```python
from build123d import *

# Parameters (mm, degrees)
SKETCH_1_R               = 27.65
SKETCH_1_R_2             = 17.65
EXTRUDE_1_DEPTH          = 167.37
CUT_EXTRUDE_1_DEPTH      = 20
CUT_EXTRUDE_START        = 147.37
CUT_EXTRUDE_2_DEPTH      = 20
CUT_EXTRUDE_4_DEPTH      = 26
CUT_EXTRUDE_4_DEPTH_BACK = 26
SKETCH_5_R               = 1.6
CUT_EXTRUDE_START_2      = 27.194163
CUT_EXTRUDE_3_DEPTH      = 2.45
CUT_EXTRUDE_5_DEPTH      = 2.45
CUT_EXTRUDE_START_3      = 27.2
CUT_EXTRUDE_6_DEPTH      = 2.45
PATTERN_CIRCULAR_2_COUNT = 4
SKETCH_8_R               = 1.6
CUT_EXTRUDE_7_DEPTH      = 32.4
PATTERN_CIRCULAR_3_COUNT = 4


with BuildPart() as part:
    # 草图1 → 凸台-拉伸1 (new body)
    with BuildSketch(Plane(origin=(0, 0, 0), x_dir=(1, 0, 0), z_dir=(0, 1, 0))):
        with Locations(Location((0, 0, 0), (0, 0, 270))):
            Circle(SKETCH_1_R)
        with Locations(Location((0, 0, 0), (0, 0, 270))):
            Circle(SKETCH_1_R_2, mode=Mode.SUBTRACT)
    extrude(amount=EXTRUDE_1_DEPTH)

    # 草图2 → 切除-拉伸1 (cut)
    with BuildSketch(Plane(origin=(0, 0, 0), x_dir=(1, 0, 0), z_dir=(0, 1, 0))):
        with BuildLine():
            Line((-27.194162977, 5), (-27.194162977, -5))
            ThreePointArc((-27.194162977, -5), (-27.65, 0), (-27.194162977, 5))
        make_face()
        with BuildLine():
            Line((27.194162977, -5), (27.194162977, 5))
            ThreePointArc((27.194162977, 5), (27.65, 0), (27.194162977, -5))
        make_face()
    extrude(amount=CUT_EXTRUDE_1_DEPTH, mode=Mode.SUBTRACT)

    # 草图3 → 切除-拉伸2 (cut)
    with BuildSketch(Plane(origin=(0, 0, 0), x_dir=(1, 0, 0), z_dir=(0, 1, 0)).offset(CUT_EXTRUDE_START)):
        with BuildLine():
            Line((-27.194162977, 5), (-27.194162977, -5))
            ThreePointArc((-27.194162977, -5), (-27.65, 0), (-27.194162977, 5))
        make_face()
        with BuildLine():
            Line((-5, -27.194162977), (5, -27.194162977))
            ThreePointArc((5, -27.194162977), (0, -27.65), (-5, -27.194162977))
        make_face()
        with BuildLine():
            Line((27.194162977, -5), (27.194162977, 5))
            ThreePointArc((27.194162977, 5), (27.65, 0), (27.194162977, -5))
        make_face()
        with BuildLine():
            Line((5, 27.194162977), (-5, 27.194162977))
            ThreePointArc((-5, 27.194162977), (0, 27.65), (5, 27.194162977))
        make_face()
    extrude(amount=CUT_EXTRUDE_2_DEPTH, mode=Mode.SUBTRACT)

    # 草图5 → 切除-拉伸4 (cut, two sides: drawn at the far end of the back side and taken through both)
    with BuildSketch(Plane.ZY.offset(-CUT_EXTRUDE_4_DEPTH_BACK)):
        with Locations((0, 5)):
            Circle(SKETCH_5_R)
    extrude(amount=CUT_EXTRUDE_4_DEPTH + CUT_EXTRUDE_4_DEPTH_BACK, mode=Mode.SUBTRACT)

    # 草图4 → 切除-拉伸3 (cut)
    with BuildSketch(Plane.ZY.offset(CUT_EXTRUDE_START_2)):
        Polygon((0, 8.233161507), (-2.8, 6.616580754), (-2.8, 3.383419246), (0, 1.766838493), (2.8, 3.383419246), (2.8, 6.616580754), align=None)
    extrude(amount=-CUT_EXTRUDE_3_DEPTH, mode=Mode.SUBTRACT)

    # 草图6 → 切除-拉伸5 (cut)
    with BuildSketch(Plane(origin=(0, 0, 0), x_dir=(0, 0, -1), z_dir=(1, 0, 0)).offset(CUT_EXTRUDE_START_2)):
        Polygon((0, 8.233161507), (-2.8, 6.616580754), (-2.8, 3.383419246), (0, 1.766838493), (2.8, 3.383419246), (2.8, 6.616580754), align=None)
    extrude(amount=-CUT_EXTRUDE_5_DEPTH, mode=Mode.SUBTRACT)

    # 草图7 → 切除-拉伸6 (cut)
    with BuildSketch(Plane(origin=(0, 0, 0), x_dir=(0, 0, -1), z_dir=(1, 0, 0)).offset(CUT_EXTRUDE_START_3)):
        Polygon((0, 165.603161507), (-2.8, 163.986580754), (-2.8, 160.753419246), (0, 159.136838493), (2.8, 160.753419246), (2.8, 163.986580754), align=None)
    cut_extrude_6 = extrude(amount=-CUT_EXTRUDE_6_DEPTH, mode=Mode.SUBTRACT)

    # 阵列(圆周)2: 切除-拉伸6 ×4 about axis
    pattern_circular_2_axis = Axis((0, 0, 0), (0, 1, 0))
    for i in range(1, PATTERN_CIRCULAR_2_COUNT):
        add(cut_extrude_6.rotate(pattern_circular_2_axis, i * 360 / PATTERN_CIRCULAR_2_COUNT), mode=Mode.SUBTRACT)

    # 草图8 → 切除-拉伸7 (cut)
    with BuildSketch(Plane(origin=(0, 0, 0), x_dir=(0, 0, -1), z_dir=(1, 0, 0))):
        with Locations(Location((0, 162.37, 0), (0, 0, 180))):
            Circle(SKETCH_8_R)
    cut_extrude_7 = extrude(amount=CUT_EXTRUDE_7_DEPTH, mode=Mode.SUBTRACT)

    # 阵列(圆周)3: 切除-拉伸7 ×4 about axis
    pattern_circular_3_axis = Axis((0, 167.37, 0), (0, -1, 0))
    for i in range(1, PATTERN_CIRCULAR_3_COUNT):
        add(cut_extrude_7.rotate(pattern_circular_3_axis, i * 360 / PATTERN_CIRCULAR_3_COUNT), mode=Mode.SUBTRACT)


solid = part.part
```
The listing builds one solid part. Answer for the finished solid, in the listing's coordinates (mm). A direction names the side the tool comes from. Round coordinates to 2 decimals unless told otherwise and drop trailing zeros. Write each loop counter-clockwise with the first axis right and the second up, starting at its lowest first coordinate (ties: lowest second). Pieces come first, ordered by that corner, then holes. Notation, with made-up numbers: (32.25, 18.5) -> (86.25, 18.5) arc R34 ccw to (86.25, 51.5) -> close; hole circle Ø1 at (2.5, -0.5). An arc over 180 degrees is marked (long way). Answer as a JSON object with one key per item and string values. Group by question number.
Q1. Determine the mould class of faces 1 (the face through (27.194, 10, 0)), 2 (the face through (-0.35, 163.93, -21.11)), 3 (the face through (21.21, 3.44, -0.35)), 4 (the face through (1.3, 161, -24.75)) for opening direction X: pulls with the +X half, pulls with the -X half, needs draft (parallel to the pull), parting line crosses it, or undercut.
Q2. Section C-C (y = 49) is taken. Write down the section's boundary in (x, z), plus the area to 3 significant figures.
Q3. Straight lines are drawn through the part: line 1 along Y through (x, z) = (20, 0); line 2 along Y through (x, z) = (0, 20.5); line 3 along Z through (x, y) = (2.5, 84.5). For each, find the intervals that lie inside material, in ascending order.
Q4. Each of these flat-tipped pins is pushed along its axis until it touches: pin 1 Ø4.5 at (x, y) = (1, 161.5) entering from +Z; pin 2 Ø1 at (x, y) = (-3, 86.5) entering from +Z; pin 3 Ø2.5 at (x, y) = (-26, 4.5) entering from +Z. Where does it stop, or does it pass through?
Q5. Section D-D (z = -10.5) is taken. Write down the section's boundary in (x, y), plus the area to 3 significant figures.
Q6. Section B-B (x = -9) is taken. Write down the section's boundary in (y, z), plus the area to 3 significant figures.
Q7. Which of the six approach directions +Z, -Z, +X, -X, +Y, -Y give full straight-line access (tool end or side, diameter ignored) to faces 5 (the face through (-1.3, 161, 24.75)), 6 (the face through (-27.194, 10, 0)), 7 (the face through (24.744, 3.6, 1.3))?
Q8. Section A-A (y = 5) is taken. Write down the section's boundary in (x, z).
Check values:
{
 "1": {"face 1": "pulls with the +X half", "face 2": "undercut", "face 3": "needs draft", "face 4": "undercut"},
 "2": {"outline": "circle Ø55.3 at (0, 0); hole circle Ø35.3 at (0, 0)", "area": "1,420 mm^2"},
 "3": {"line 1": "0 to 3.4, 6.6 to 160.77, 163.97 to 167.37", "line 2": "0 to 160.77, 163.97 to 167.37", "line 3": "-27.54 to -17.47, 17.47 to 27.54"},
 "4": {"pin 1": "z = 27.19", "pin 2": "z = 27.54", "pin 3": "z = 12.33"},
 "5": {"outline": "(-25.58, 0) -> (-14.19, 0) -> (-14.19, 167.37) -> (-25.58, 167.37) -> close; (14.19, 0) -> (25.58, 0) -> (25.58, 167.37) -> (14.19, 167.37) -> close", "area": "3,810 mm^2"},
 "6": {"outline": "(0, -26.14) -> (167.37, -26.14) -> (167.37, -15.18) -> (0, -15.18) -> close; (0, 15.18) -> (167.37, 15.18) -> (167.37, 26.14) -> (0, 26.14) -> close", "area": "3,670 mm^2"},
 "7": {"face 5": "+Z", "face 6": "+Z, -Z, -X, -Y", "face 7": "+X"},
 "8": {"outline": "(-27.19, -5) arc R27.65 ccw to (27.19, -5) -> (27.19, -2.8) -> (24.74, -2.8) -> (24.74, -1.6) -> (17.58, -1.6) arc R17.65 cw to (-17.58, -1.6) -> (-24.74, -1.6) -> (-24.74, -2.8) -> (-27.19, -2.8) -> close; (-27.19, 2.8) -> (-24.74, 2.8) -> (-24.74, 1.6) -> (-17.58, 1.6) arc R17.65 cw to (17.58, 1.6) -> (24.74, 1.6) -> (24.74, 2.8) -> (27.19, 2.8) -> (27.19, 5) arc R27.65 ccw to (-27.19, 5) -> close"}
}
